Can you work these out from the model? Positions are in its coordinate system, mm. A direction names the side the tool comes from. Coordinates: 2 decimals unless noted, no trailing zeros. Order: outer loops, then holes, each group sorted by start corner. A loop starts at its lowest first (then second) coordinate and runs counter-clockwise, first axis right, second up. Notation, with made-up numbers: (42.25, 21) - (101.25, 21) arc R28 ccw to (101.25, 40) - close; hole circle Ø1 at (63, 87.25). An arc over 180 degrees is marked (long way). Use a Markdown table: item, result. Add a question column.
(1) I want a section at C-C (z = 18). List the corners of the cut face in (x, y) for me, and give its area (3 significant figures).
(2) I want a section at D-D (z = -11). List the corners of the cut face in (x, y) for me.
(3) We'd pull the mould along Z, two halves only. Please class faces 4 (the cylindrical face through (19.752, -3.324, 16.819)), 5 (the flat face through (-21, 5.461, 0)), 6 (the flat face through (13.2, 8.5, -27.534)): pulls with the +Z half, pulls with the -Z half, needs draft (parallel to the pull), parting line crosses it, or undercut.
(4) I want a section at A-A (z = -18). List the corners of the cut face in (x, y) for me (1 decimal), and give its area (3 significant figures).
(5) I want a section at B-B (x = 37). List the corners of the cut face in (y, z) for me, and give its area (3 significant figures).
(6) If I drill on L1, parallel to Z at x = 22, y = 9; L2, parallel to X at y = -6, z = -24; L3, parallel to Y at x = 36, z = 15.5, over which ranges is the centre line in solid material (lowest first)? Write a range as [from, to].
(7) On a 3-axis mill with a long thin cutter (end or side, diameter ignored), from which of +Z, -Z, +X, -X, +Y, -Y can I reach the whole of each face in a straight line? I mean faces 1 (the flat face through (56, 5, -14.072)), 2 (the flat face through (32, 14.288, -2)), 3 (the cylindrical face through (-11.326, -6.187, -1.374)). Say none if no direction works.
(8) For pin 1 Ø5.5 at (y, z) = (-7.92, -16.69) entering from +X; pin 2 Ø2 at (y, z) = (-11, -12) entering from -X; pin 3 Ø8 at (y, z) = (7, -13) entering from -X; pin 4 Ø10 at (x, y) = (-5.5, -4) entering from +Z, each with a flat end and sliding along its axis, tell me the tip position at first contact or that it passes through.
```python
from build123d import *

# Parameters (mm, degrees)
SKETCH1_W          = 50.8
SKETCH1_H          = 28.575
EXTRUDE1_DEPTH     = 65.8368
LPATTERN1_COUNT    = 2
LPATTERN1_PITCH    = 46.99
SKETCH5_R          = 13.5001
EXTRUDE2_DEPTH     = 5.969
SKETCH6_W          = 6.3373
SKETCH6_H          = 16.891
CUT_EXTRUDE4_DEPTH = 30.48
HOLE1_D            = 7.137
HOLE1_DEPTH        = 65.8368
HOLE2_D            = 7.137
HOLE2_DEPTH        = 28.575


with BuildPart() as part:
    # Sketch1 → Extrude1 (new body)
    with BuildSketch(Plane(origin=(0, 0, 0), x_dir=(0, 0, -1), z_dir=(1, 0, 0))):
        with Locations((2.3876, 0)):
            Rectangle(SKETCH1_W, SKETCH1_H)
    extrude(amount=EXTRUDE1_DEPTH)

    # S2D0002 → Cut-Revolve1 (revolve, cut)
    with BuildSketch(Plane(origin=(0, 4.7625, 0), x_dir=(-1, 0, 0), z_dir=(0, 1, 0)), mode=Mode.PRIVATE) as cut_revolve1_sk:
        Polygon((-14.5415, -27.5336), (-18.161, -27.5336), (-18.161, -27.7876), (-9.525, -27.7876), (-9.525, -14.0716), (-13.9446, -14.0716), (-13.9446, -26.9113), (-14.5415, -27.5082), align=None)
    cut_revolve1 = revolve(cut_revolve1_sk.sketch.rotate(Axis((9.525, 4.7625, -19.13842003), (0, 0, 1)), 180), axis=Axis((9.525, 4.7625, -19.13842003), (0, 0, 1)), mode=Mode.SUBTRACT)  # turned: the seam where the file's is

    # LPattern1: Cut-Revolve1 ×2
    with Locations(*[(i * LPATTERN1_PITCH, 0, 0) for i in range(1, LPATTERN1_COUNT)]):
        add(cut_revolve1, mode=Mode.SUBTRACT)

    # Sketch5 → Extrude2 (add)
    with BuildSketch(Plane.ZY):
        Circle(SKETCH5_R)
    extrude(amount=EXTRUDE2_DEPTH)

    # Sketch6 → Revolve1 (revolve)
    with BuildSketch(Plane(origin=(0, 0, 0), x_dir=(0, 0, 1), z_dir=(0, -1, 0)), mode=Mode.PRIVATE) as revolve1_sk:
        with Locations((-3.16865, 14.4145)):
            Rectangle(SKETCH6_W, SKETCH6_H)
    revolve(revolve1_sk.sketch.rotate(Axis((5.754582971, 0, 0), (-1, 0, 0)), 180), axis=Axis((5.754582971, 0, 0), (-1, 0, 0)))  # turned: the seam where the file's is

    # S2D0001 → Cut-Revolve4 (revolve, cut)
    with BuildSketch(Plane(origin=(-18.511260017, 3.2639, 0), x_dir=(0, 1, 0), z_dir=(0, 0, 1)), mode=Mode.PRIVATE) as cut_revolve4_sk:
        Polygon((-0.7493, 2.984923177), (-0.7493, -11.653260017), (-3.2639, -13.16418413), (-3.2639, 4.348739983), (0.0381, 4.348739983), align=None)
    revolve(cut_revolve4_sk.sketch.rotate(Axis((0, 0, 0), (-1, 0, 0)), 90), axis=Axis((0, 0, 0), (-1, 0, 0)), mode=Mode.SUBTRACT)  # turned: the seam where the file's is

    # Sketch8 → Cut-Revolve5 (revolve, cut)
    with BuildSketch(Plane(origin=(0, 0, 0), x_dir=(0, 0, -1), z_dir=(0, 1, 0)), mode=Mode.PRIVATE) as cut_revolve5_sk:
        with BuildLine():
            Line((-6.3373, 16.5354), (-6.096, 17.2974))
            Line((-6.096, 17.2974), (-6.096, 21.844))
            ThreePointArc((-6.096, 21.844), (-5.995678675, 22.387796865), (-5.707922533, 22.86))
            Line((-5.707922533, 22.86), (-6.3373, 22.86))
            Line((-6.3373, 22.86), (-6.3373, 16.5354))
        make_face()
    revolve(cut_revolve5_sk.sketch.rotate(Axis((-12.65936, 0, 0), (-1, 0, 0)), 180), axis=Axis((-12.65936, 0, 0), (-1, 0, 0)), mode=Mode.SUBTRACT)  # turned: the seam where the file's is

    # Sketch12 → Cut-Extrude4 (cut, symmetric)
    with BuildSketch(Plane(origin=(0, 0, 0), x_dir=(0, -1, 0), z_dir=(0, 0, -1))):
        Polygon((5.461, 22.86), (5.461, 18.0848), (6.096, 17.4498), (6.096, 22.86), align=None)
        Polygon((-5.461, 22.86), (-5.461, 18.0848), (-6.096, 17.4498), (-6.096, 22.86), align=None)
    extrude(amount=CUT_EXTRUDE4_DEPTH, both=True, mode=Mode.SUBTRACT)

    # Hole1
    with Locations(Plane.ZY):
        with Locations((-16.6878, -7.9248), (16.6624, 7.9502)):
            Hole(HOLE1_D / 2, depth=HOLE1_DEPTH)

    # Hole2
    with Locations(Plane(origin=(0, 14.2875, 0), x_dir=(-1, 0, 0), z_dir=(0, 1, 0))):
        with Locations((-23.3172, -16.6878), (-23.3172, 16.6624)):
            Hole(HOLE2_D / 2, depth=HOLE2_DEPTH)


solid = part.part
```
Answers follow:
| question | item | result |
|---|---|---|
| 1 | outline | (0, -14.29) - (20.01, -14.29) - (20.01, 4.64) - (0, 4.64) - close; (0, 11.26) - (20.01, 11.26) - (20.01, 14.29) - (0, 14.29) - close; (26.63, -14.29) - (65.84, -14.29) - (65.84, 4.64) - (26.63, 4.64) - close; (26.63, 11.26) - (65.84, 11.26) - (65.84, 14.29) - (26.63, 14.29) - close |
| 1 | area | 1,300 mm² |
| 2 | outline | (-5.97, -7.83) - (0, -7.83) - (0, -14.29) - (65.84, -14.29) - (65.84, 14.29) - (0, 14.29) - (0, 7.83) - (-5.97, 7.83) - close |
| 3 | face 4 | undercut |
| 3 | face 5 | needs draft |
| 3 | face 6 | pulls with the -Z half |
| 4 | outline | (0, -14.3) - (20, -14.3) - (20, -11.2) - (0, -11.2) - close; (0, -4.6) - (20, -4.6) - (20, 14.3) - (0, 14.3) - close; (26.6, -14.3) - (65.8, -14.3) - (65.8, -11.2) - (26.6, -11.2) - close; (26.6, -4.6) - (65.8, -4.6) - (65.8, 14.3) - (26.6, 14.3) - close; hole circle Ø8.8 at (9.5, 4.8); hole circle Ø8.8 at (56.5, 4.8) |
| 4 | area | 1,180 mm² |
| 5 | outline | (-14.29, -27.79) - (14.29, -27.79) - (14.29, 23.01) - (-14.29, 23.01) - close; hole circle Ø7.14 at (-7.92, -16.69); hole circle Ø7.14 at (7.95, 16.66) |
| 5 | area | 1,370 mm² |
| 6 | L1 | z = [-27.79, -20], [-13.37, 13.25], [20.07, 23.01] |
| 6 | L2 | x = [0, 65.84] |
| 6 | L3 | y = [-14.29, 4.58], [11.32, 14.29] |
| 7 | face 1 | -Z |
| 7 | face 2 | +Z, -Z, +X, -X, +Y |
| 7 | face 3 | -X |
| 8 | pin 1 | passes through |
| 8 | pin 2 | stops at x = 0 |
| 8 | pin 3 | stops at x = -5.97 |
| 8 | pin 4 | stops at z = 13.5 |
